from build123d import *

# Parameters (mm, degrees)
F1_DEPTH = 25
F0_W     = 100
F0_H     = 100
F2_DEPTH = 3


with BuildPart() as f1:
    # F0 (on Top) → F1 (new body)
    with BuildSketch(Plane.XY):
        with BuildLine():
            ThreePointArc((-72, 64.9100722949), (-74.1114641858, 66.7425764269), (-75, 69.3933982822))
            Line((-75, 69.3933982822), (-75, -69.3933982822))
            ThreePointArc((-75, -69.3933982822), (-74.1114641858, -66.7425764269), (-72, -64.9100722949))
            Line((-72, -64.9100722949), (-72, -61.9100722949))
            Line((-72, -61.9100722949), (-72, 61.9100722949))
            Line((-72, 61.9100722949), (-72, 64.9100722949))
        make_face()
        with BuildLine():
            Line((-61.9100722949, 72), (-64.9100722949, 72))
            ThreePointArc((-64.9100722949, 72), (-65.9405713869, 65.9405713869), (-72, 64.9100722949))
            Line((-72, 64.9100722949), (-72, 61.9100722949))
            ThreePointArc((-72, 61.9100722949), (-64.0021028341, 64.0021028341), (-61.9100722949, 72))
        make_face()
        with BuildLine():
            Line((69.3933982822, 75), (-69.3933982822, 75))
            ThreePointArc((-69.3933982822, 75), (-66.7425764269, 74.1114641858), (-64.9100722949, 72))
            Line((-64.9100722949, 72), (-61.9100722949, 72))
            Line((-61.9100722949, 72), (61.9100722949, 72))
            Line((61.9100722949, 72), (64.9100722949, 72))
            ThreePointArc((64.9100722949, 72), (66.7425764269, 74.1114641858), (69.3933982822, 75))
        make_face()
        with BuildLine():
            ThreePointArc((72, 64.9100722949), (65.9405713869, 65.9405713869), (64.9100722949, 72))
            Line((64.9100722949, 72), (61.9100722949, 72))
            ThreePointArc((61.9100722949, 72), (64.0021028341, 64.0021028341), (72, 61.9100722949))
            Line((72, 61.9100722949), (72, 64.9100722949))
        make_face()
        with BuildLine():
            ThreePointArc((75, 69.3933982822), (74.1114641858, 66.7425764269), (72, 64.9100722949))
            Line((72, 64.9100722949), (72, 61.9100722949))
            Line((72, 61.9100722949), (72, -61.9100722949))
            Line((72, -61.9100722949), (72, -64.9100722949))
            ThreePointArc((72, -64.9100722949), (74.1114641858, -66.7425764269), (75, -69.3933982822))
            Line((75, -69.3933982822), (75, 69.3933982822))
        make_face()
        with BuildLine():
            Line((72, -64.9100722949), (72, -61.9100722949))
            ThreePointArc((72, -61.9100722949), (64.0021028341, -64.0021028341), (61.9100722949, -72))
            Line((61.9100722949, -72), (64.9100722949, -72))
            ThreePointArc((64.9100722949, -72), (65.9405713869, -65.9405713869), (72, -64.9100722949))
        make_face()
        with BuildLine():
            Line((-61.9100722949, -72), (-64.9100722949, -72))
            ThreePointArc((-64.9100722949, -72), (-66.7425764269, -74.1114641858), (-69.3933982822, -75))
            Line((-69.3933982822, -75), (69.3933982822, -75))
            ThreePointArc((69.3933982822, -75), (66.7425764269, -74.1114641858), (64.9100722949, -72))
            Line((64.9100722949, -72), (61.9100722949, -72))
            Line((61.9100722949, -72), (-61.9100722949, -72))
        make_face()
        with BuildLine():
            Line((-72, -61.9100722949), (-72, -64.9100722949))
            ThreePointArc((-72, -64.9100722949), (-65.9405713869, -65.9405713869), (-64.9100722949, -72))
            Line((-64.9100722949, -72), (-61.9100722949, -72))
            ThreePointArc((-61.9100722949, -72), (-63.8192510434, -63.8192510434), (-72, -61.9100722949))
        make_face()
    extrude(amount=F1_DEPTH)

    # F0 (on Top) → F2 (join)
    with BuildSketch(Plane.XY):
        with BuildLine():
            Line((61.9100722949, 72), (-61.9100722949, 72))
            ThreePointArc((-61.9100722949, 72), (-64.0021028341, 64.0021028341), (-72, 61.9100722949))
            Line((-72, 61.9100722949), (-72, -61.9100722949))
            ThreePointArc((-72, -61.9100722949), (-63.8192510434, -63.8192510434), (-61.9100722949, -72))
            Line((-61.9100722949, -72), (61.9100722949, -72))
            ThreePointArc((61.9100722949, -72), (64.0021028341, -64.0021028341), (72, -61.9100722949))
            Line((72, -61.9100722949), (72, 61.9100722949))
            ThreePointArc((72, 61.9100722949), (64.0021028341, 64.0021028341), (61.9100722949, 72))
        make_face()
        Rectangle(F0_W, F0_H, mode=Mode.SUBTRACT)
    extrude(amount=F2_DEPTH)


solid = f1.part
Read the model definition and answer for the solid it produces. Units are mm, in the model's axes. A direction names the side the tool comes from. Give positions to 0.01 mm unless a question says otherwise; leave off trailing zeros. Write each loop counter-clockwise with the first axis right and the second up, starting at its lowest first coordinate (ties: lowest second). Pieces come first, ordered by that corner, then holes. Notation, with made-up numbers: (70.5, 81.25) - (88.5, 81.25) arc R25 cw to (88.5, 99.25) - close; hole circle Ø3 at (-32, 80.5). An arc over 180 degrees is marked (long way). Answer in a Markdown table with one row per item. Add a question column.
Item 1: Find the intervals of material crossed by L1, parallel to Y at x = 23.5, z = 5; L2, parallel to X at y = 67, z = 10.5, in increasing order.
Item 2: A tool of negligible diameter and unlimited length cuts with its end or side. For faces 1 (the face through (-75, 1, 12)), 2 (the face through (-72, -1, 14)), from which of +Z, -Z, +X, -X, +Y, -Y can it reach the whole face along a straight path? Write none if from no direction.
Item 3: Section D-D, the plane x = -58 is taken. Write down the section's boundary in (y, z).
Item 4: Determine the mould class of faces 3 (the face through (-1, 51, 0)), 4 (the face through (1, -72, 14)), 5 (the face through (63.917, 64.089, 13.846)), 6 (the face through (-1, -75, 12)) for opening direction Y: pulls with the +Y half, pulls with the -Y half, needs draft (parallel to the pull), parting line crosses it, or undercut.
Item 5: Section C-C, the plane z = 19.5 is taken. Write down the section's boundary in (x, y), and give its area (3 significant figures).
Item 6: Section A-A, the plane x = 41.5 is taken. Write down the section's boundary in (y, z), and give its area (3 significant figures).
Recorded:
| question | item | result |
|---|---|---|
| 1 | L1 | y = -75 to -72, 72 to 75 |
| 1 | L2 | x = -75 to -74.27, -65.12 to -62.1, 62.1 to 65.12, 74.27 to 75 |
| 2 | face 1 | +Z, -Z, -X, +Y, -Y |
| 2 | face 2 | +Z |
| 3 | outline | (-75, 0) - (75, 0) - (75, 25) - (72, 25) - (72, 3) - (-72, 3) - (-72, 25) - (-75, 25) - close |
| 4 | face 3 | needs draft |
| 4 | face 4 | undercut |
| 4 | face 5 | undercut |
| 4 | face 6 | pulls with the -Y half |
| 5 | outline | (-75, -69.39) arc R5.31 cw (long way) to (-69.39, -75) - (69.39, -75) arc R5.31 cw (long way) to (75, -69.39) - (75, 69.39) arc R5.31 cw (long way) to (69.39, 75) - (-69.39, 75) arc R5.31 cw (long way) to (-75, 69.39) - close; hole (-72, -61.91) arc R7.96 cw to (-61.91, -72) - (61.91, -72) arc R8.18 cw to (72, -61.91) - (72, 61.91) arc R8.18 cw to (61.91, 72) - (-61.91, 72) arc R8.18 cw to (-72, 61.91) - close |
| 5 | area | 1,760 mm2 |
| 6 | outline | (-75, 0) - (-50, 0) - (-50, 3) - (-72, 3) - (-72, 25) - (-75, 25) - close; (50, 0) - (75, 0) - (75, 25) - (72, 25) - (72, 3) - (50, 3) - close |
| 6 | area | 282 mm2 |
